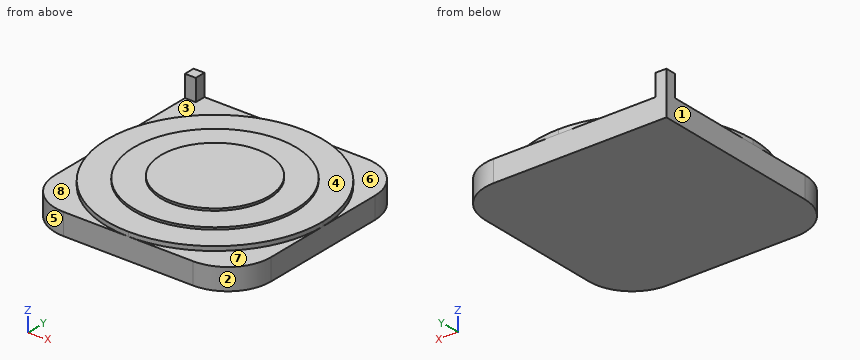
from build123d import *

# Parameters (mm, degrees)
F1_DEPTH = 2.54
F0_W     = 1.27
F0_H     = 1.27
F2_DEPTH = 3.048
F3_DEPTH = 5.08
F4_DEPTH = 3.302
F5_DEPTH = 3.556
F6_R     = 5.08


with BuildPart() as f1:
    # F0 (on Top) → F1 (new body)
    with BuildSketch(Plane.XY):
        with BuildLine():
            Line((0, 12.7), (0, 0))
            Line((0, 0), (12.7, 0))
            ThreePointArc((12.7, 0), (3.7197438789, 3.7197438789), (0, 12.7))
        make_face()
    extrude(amount=F1_DEPTH)



with BuildPart() as f1b:
    # F0 (on Top) → F1, piece 2 (new body)
    with BuildSketch(Plane.XY):
        with Locations((0.635, 24.765)):
            Rectangle(F0_W, F0_H)
        with BuildLine():
            Line((0, 24.13), (0, 12.7))
            ThreePointArc((0, 12.7), (3.7197438789, 21.6802561211), (12.7, 25.4))
            Line((12.7, 25.4), (1.27, 25.4))
            Line((1.27, 25.4), (1.27, 24.13))
            Line((1.27, 24.13), (0, 24.13))
        make_face()
    extrude(amount=F1_DEPTH)


with BuildPart() as f1c:
    # F0 (on Top) → F1, piece 3 (new body)
    with BuildSketch(Plane.XY):
        with BuildLine():
            Line((25.4, 25.4), (12.7, 25.4))
            ThreePointArc((12.7, 25.4), (21.6802561211, 21.6802561211), (25.4, 12.7))
            Line((25.4, 12.7), (25.4, 25.4))
        make_face()
    extrude(amount=F1_DEPTH)


with BuildPart() as f1d:
    # F0 (on Top) → F1, piece 4 (new body)
    with BuildSketch(Plane.XY):
        with BuildLine():
            ThreePointArc((25.4, 12.7), (21.6802561211, 3.7197438789), (12.7, 0))
            Line((12.7, 0), (25.4, 0))
            Line((25.4, 0), (25.4, 12.7))
        make_face()
    extrude(amount=F1_DEPTH)


with BuildPart() as f1_1:
    add(f1.part)

    add(f1b.part)  # F2 merges F1b

    add(f1c.part)  # F2 merges F1c

    add(f1d.part)  # F2 merges F1d
    # F0 (on Top) → F2 (join)
    with BuildSketch(Plane.XY):
        with BuildLine():
            Line((3.175, 12.7), (0, 12.7))
            ThreePointArc((0, 12.7), (3.7197438789, 3.7197438789), (12.7, 0))
            Line((12.7, 0), (12.7, 3.175))
            ThreePointArc((12.7, 3.175), (5.9648079092, 5.9648079092), (3.175, 12.7))
        make_face()
        with BuildLine():
            ThreePointArc((25.4, 12.7), (21.6802561211, 21.6802561211), (12.7, 25.4))
            Line((12.7, 25.4), (12.7, 22.225))
            ThreePointArc((12.7, 22.225), (19.4351920908, 19.4351920908), (22.225, 12.7))
            Line((22.225, 12.7), (25.4, 12.7))
        make_face()
        with BuildLine():
            Line((12.7, 3.175), (12.7, 0))
            ThreePointArc((12.7, 0), (21.6802561211, 3.7197438789), (25.4, 12.7))
            Line((25.4, 12.7), (22.225, 12.7))
            ThreePointArc((22.225, 12.7), (19.4351920908, 5.9648079092), (12.7, 3.175))
        make_face()
        with BuildLine():
            ThreePointArc((12.7, 25.4), (3.7197438789, 21.6802561211), (0, 12.7))
            Line((0, 12.7), (3.175, 12.7))
            ThreePointArc((3.175, 12.7), (5.9648079092, 19.4351920908), (12.7, 22.225))
            Line((12.7, 22.225), (12.7, 25.4))
        make_face()
    extrude(amount=F2_DEPTH)

    # F0 (on Top) → F3 (join)
    with BuildSketch(Plane.XY):
        with Locations((0.635, 24.765)):
            Rectangle(F0_W, F0_H)
    extrude(amount=F3_DEPTH)

    # F0 (on Top) → F4 (join)
    with BuildSketch(Plane.XY):
        with BuildLine():
            ThreePointArc((12.7, 22.225), (5.9648079092, 19.4351920908), (3.175, 12.7))
            Line((3.175, 12.7), (6.35, 12.7))
            ThreePointArc((6.35, 12.7), (8.2098719395, 17.1901280605), (12.7, 19.05))
            Line((12.7, 19.05), (12.7, 22.225))
        make_face()
        with BuildLine():
            ThreePointArc((22.225, 12.7), (19.4351920908, 19.4351920908), (12.7, 22.225))
            Line((12.7, 22.225), (12.7, 19.05))
            ThreePointArc((12.7, 19.05), (17.1901280605, 17.1901280605), (19.05, 12.7))
            Line((19.05, 12.7), (22.225, 12.7))
        make_face()
        with BuildLine():
            Line((6.35, 12.7), (3.175, 12.7))
            ThreePointArc((3.175, 12.7), (5.9648079092, 5.9648079092), (12.7, 3.175))
            Line((12.7, 3.175), (12.7, 6.35))
            ThreePointArc((12.7, 6.35), (8.2098719395, 8.2098719395), (6.35, 12.7))
        make_face()
        with BuildLine():
            Line((12.7, 6.35), (12.7, 3.175))
            ThreePointArc((12.7, 3.175), (19.4351920908, 5.9648079092), (22.225, 12.7))
            Line((22.225, 12.7), (19.05, 12.7))
            ThreePointArc((19.05, 12.7), (17.1901280605, 8.2098719395), (12.7, 6.35))
        make_face()
    extrude(amount=F4_DEPTH)

    # F0 (on Top) → F5 (join)
    with BuildSketch(Plane.XY):
        with BuildLine():
            ThreePointArc((12.7, 19.05), (8.2098719395, 17.1901280605), (6.35, 12.7))
            Line((6.35, 12.7), (12.7, 12.7))
            Line((12.7, 12.7), (12.7, 19.05))
        make_face()
        with BuildLine():
            Line((12.7, 12.7), (6.35, 12.7))
            ThreePointArc((6.35, 12.7), (8.2098719395, 8.2098719395), (12.7, 6.35))
            Line((12.7, 6.35), (12.7, 12.7))
        make_face()
        with BuildLine():
            Line((12.7, 19.05), (12.7, 12.7))
            Line((12.7, 12.7), (19.05, 12.7))
            ThreePointArc((19.05, 12.7), (17.1901280605, 17.1901280605), (12.7, 19.05))
        make_face()
        with BuildLine():
            Line((12.7, 12.7), (12.7, 6.35))
            ThreePointArc((12.7, 6.35), (17.1901280605, 8.2098719395), (19.05, 12.7))
            Line((19.05, 12.7), (12.7, 12.7))
        make_face()
    extrude(amount=F5_DEPTH)

    # F6
    f6_edges = [f1_1.edges().sort_by_distance(p)[0] for p in [
        (0, 0, 1.27),
        (25.4, 25.4, 1.27),
        (25.4, 0, 1.27),
    ]]
    fillet(f6_edges, radius=F6_R)


solid = f1_1.part
Work out the finished part from the listing and answer in its coordinate system (mm). Face numbers are marked on the shaded views. A direction names the side the tool comes from. Round coordinates to 2 decimals unless told otherwise and drop trailing zeros. Write each loop counter-clockwise with the first axis right and the second up, starting at its lowest first coordinate (ties: lowest second). Pieces come first, ordered by that corner, then holes. Notation, with made-up numbers: (-2.5, 66) -> (20.5, 66) arc R36 cw to (20.5, 103) -> close; hole circle Ø2 at (-29, 80). An arc over 180 degrees is marked (long way). Answer as CSV lines item,"result". Start each with the question number.
(1) The part is cut by section C-C, the plane x = 7. Give the vertices of the cut face in (y, z), then the cut area to 3 significant figures.
(2) The part is cut by section D-D, the plane y = 2. Give the vertices of the cut face in (x, z), then the cut area to 3 significant figures.
(3) Find the intervals of material crossed by probe 1 along Z at (x, y) = (11, 2.5); probe 2 along Z at (x, y) = (7, 11.25); probe 3 along Y at (x, z) = (1, 3.1), in increasing order.
(4) The part is cut by section A-A, the plane z = 0.9. Give the vertices of the cut face in (x, y).
(5) A tool of negligible diameter and unlimited length cuts with its end or side. For the marked faces 4, 5, 6, 7 and 8, from which of +Z, -Z, +X, -X, +Y, -Y can it reach the whole face along a straight path? Write none if from no direction.
(6) The part is cut by section B-B, the plane y = 18. Give the vertices of the cut face in (x, z), then the cut area to 3 significant figures.
(7) The mould has two halves that part along Y. Classify the marked faces 1, 2 and 3: +Y half, -Y half, draft (parallel to the pull), parting line (faces both ways), or undercut.
(8) Each of these flat-tipped pins is pushed along its axis until it touches: pin 1 (5 mm diameter, centred on x = 22.5, y = 10, fed in from +Z); pin 2 (10 mm diameter, centred on x = 22, y = 7, fed in from +Z); pin 3 (14 mm diameter, centred on x = 3, y = 17.5, fed in from +Z). Where does it stop, or does it pass through?
Output values:
1,outline,"(0, 0) -> (25.4, 0) -> (25.4, 2.54) -> (24.05, 2.54) -> (24.05, 3.05) -> (20.33, 3.05) -> (20.33, 3.3) -> (15.5, 3.3) -> (15.5, 3.56) -> (9.9, 3.56) -> (9.9, 3.3) -> (5.07, 3.3) -> (5.07, 3.05) -> (1.35, 3.05) -> (1.35, 2.54) -> (0, 2.54) -> close"
1,area,"81.3 mm²"
2,outline,"(1.04, 0) -> (24.36, 0) -> (24.36, 2.54) -> (19.54, 2.54) -> (19.54, 3.05) -> (5.86, 3.05) -> (5.86, 2.54) -> (1.04, 2.54) -> close"
2,area,"66.2 mm²"
3,probe 1,"z = 0 to 3.05"
3,probe 2,"z = 0 to 3.56"
3,probe 3,"y = 24.13 to 25.4"
4,outline,"(0, 5.08) arc R5.08 ccw to (5.08, 0) -> (20.32, 0) arc R5.08 ccw to (25.4, 5.08) -> (25.4, 20.32) arc R5.08 ccw to (20.32, 25.4) -> (0, 25.4) -> close"
5,face 4,"+Z"
5,face 5,"+Z, -Z, -X, -Y"
5,face 6,"+Z, +X, +Y"
5,face 7,"+Z, +X, -Y"
5,face 8,"+Z, -X, -Y"
6,outline,"(0, 0) -> (25.4, 0) -> (25.4, 2.54) -> (24.24, 2.54) -> (24.24, 3.05) -> (20.61, 3.05) -> (20.61, 3.3) -> (16.2, 3.3) -> (16.2, 3.56) -> (9.2, 3.56) -> (9.2, 3.3) -> (4.79, 3.3) -> (4.79, 3.05) -> (1.16, 3.05) -> (1.16, 2.54) -> (0, 2.54) -> close"
6,area,"82.0 mm²"
7,face 1,"draft"
7,face 2,"-Y half"
7,face 3,"undercut"
8,pin 1,"stops at z = 3.3"
8,pin 2,"stops at z = 3.56"
8,pin 3,"stops at z = 5.08"
